Read the model definition and answer for the solid it produces. Units are mm, in the model's axes. Face numbers are marked on the shaded views. Coordinates: 2 decimals unless noted, no trailing zeros. Write each loop counter-clockwise with the first axis right and the second up, starting at its lowest first coordinate (ties: lowest second). Pieces come first, ordered by that corner, then holes.
Item 1: Section C-C (z = 3.5) is taken. Give the vertices of the cut face in (x, y), then the cut area to 3 significant figures.
Item 2: Section A-A (y = 0) is taken. Give the vertices of the cut face in (x, z), then the cut area to 3 significant figures.
Item 3: Determine the mould class of the marked faces 1 and 2 for opening direction X: released by +X, released by -X, zero draft, split by the parting line, or undercut.
Item 4: Each of these flat-tipped pins is pushed along its axis until it touches: P1, Ø2, axis at x = 7, z = 5, coming from the +Y side; P2, Ø10, axis at y = 14.2, z = 11.11, coming from the -X side; P3, Ø1.5, axis at y = 2.5, z = 14, coming from the -X side. Where does it stop, or does it pass through?
Item 5: Straight lines are drawn through the part: probe 1 along X at (y, z) = (1, 17); probe 2 along X at (y, z) = (-36.5, 10); probe 3 along Y at (x, z) = (-24.5, 10.5). For each, find the intervals that lie inside material, in ascending order.
from build123d import *

# Parameters (mm, degrees)
SKETCH1_R               = 50.8
SKETCH1_R_2             = 49.6697
BOSS_EXTRUDE1_DEPTH     = 23.3299
CUT_EXTRUDE1_DEPTH      = 76.535185404
CUT_EXTRUDE1_DEPTH_BACK = 76.535185404
SKETCH2_R               = 3.175


with BuildPart() as part:
    # Sketch1 → Boss-Extrude1 (new, symmetric)
    with BuildSketch(Plane.XY):
        Circle(SKETCH1_R)
        Circle(SKETCH1_R_2, mode=Mode.SUBTRACT)
    extrude(amount=BOSS_EXTRUDE1_DEPTH, both=True)

    # Sketch2 → Cut-Extrude1 (cut, two sides: drawn at the far end of the back side and taken through both)
    with BuildSketch(Plane(origin=(0, 0, 0), x_dir=(0, 0, -1), z_dir=(1, 0, 0)).offset(-CUT_EXTRUDE1_DEPTH_BACK)):
        with Locations((-11.1125, 14.20368)):
            Circle(SKETCH2_R)
        with Locations((11.1125, 14.20368)):
            Circle(SKETCH2_R)
    extrude(amount=CUT_EXTRUDE1_DEPTH + CUT_EXTRUDE1_DEPTH_BACK, mode=Mode.SUBTRACT)


solid = part.part
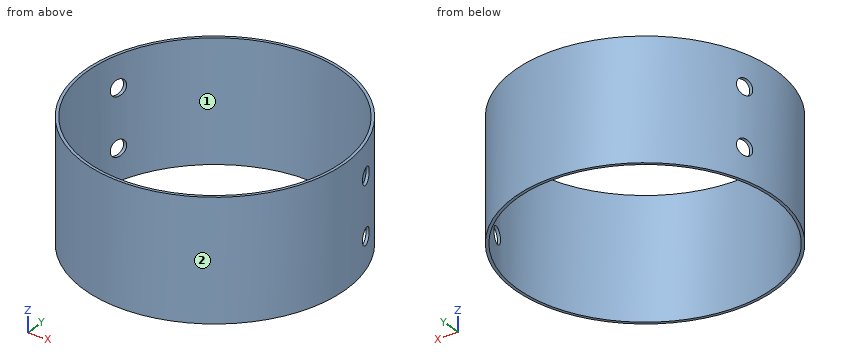
Established:
1. outline: circle Ø101.6 at (0, 0); hole circle Ø99.34 at (0, 0)
1. area: 357 mm2
2. outline: (-50.8, -23.33) - (-49.67, -23.33) - (-49.67, 23.33) - (-50.8, 23.33) - close; (49.67, -23.33) - (50.8, -23.33) - (50.8, 23.33) - (49.67, 23.33) - close
2. area: 105 mm2
3. face 1: undercut
3. face 2: split by the parting line
4. P1: stops at y = 50.44
4. P2: stops at x = -49.96
4. P3: stops at x = -50.77
5. probe 1: x = -50.79 to -49.66, 49.66 to 50.79
5. probe 2: x = -35.33 to -33.69, 33.69 to 35.33
5. probe 3: y = -44.5 to -43.21, 43.21 to 44.5
